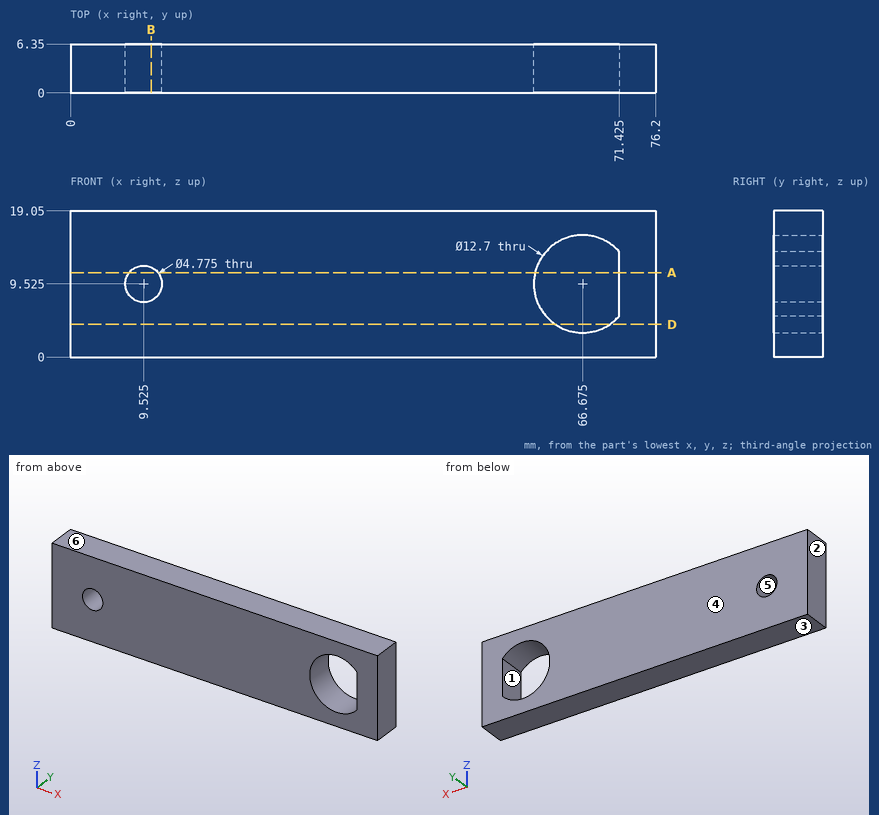
Design review of the part shown in the three views and the two pictorial views. Dimensions are in mm from the part's minimum x, y and z. A direction names the side the tool comes from. Round coordinates to 2 decimals unless told otherwise and drop trailing zeros. Loops run counter-clockwise (first coordinate to the right, second up) from the corner with the lowest first, then second, coordinate; pieces in that order, holes last. Notation, with made-up numbers: (66.25, -8) -> (103.25, -8) arc R23 ccw to (103.25, 11) -> close; hole circle Ø3 at (71.5, 7.25). An arc over 180 degrees is marked (long way). Return JSON: item names as keys, results as strings.
(1) For line 1 (X direction, y = 1.75, z = 9.75) (1 decimal); line 2 (X direction, y = 3.75, z = 7.5) (1 decimal); line 3 (X direction, y = 2.5, z = 5.75) (1 decimal), list the stretches that pass through material, from the lowest coordinate up.
Solved:
{"line 1": "0 to 7.1, 11.9 to 60.3, 71.4 to 76.2", "line 2": "0 to 8.3, 10.8 to 60.7, 71.4 to 76.2", "line 3": "0 to 61.6, 71.4 to 76.2"}
(2) Add section B-B on x = 10.5. Write out the cut boundary in (y, z), plus the area to 3 significant figures.
Solved:
{"outline": "(0, 0) -> (6.35, 0) -> (6.35, 7.35) -> (0, 7.35) -> close; (0, 11.7) -> (6.35, 11.7) -> (6.35, 19.05) -> (0, 19.05) -> close", "area": "93.3 mm2"}
(3) The part is to be moulded in two halves that separate along Z. For the marked faces 3, 4, 5 and 6, say which applies: released by +Z, released by -Z, zero draft, split by the parting line, or undercut.
Solved:
{"face 3": "released by -Z", "face 4": "zero draft", "face 5": "undercut", "face 6": "released by +Z"}
(4) Add section A-A on z = 11. State how many separate pieces and enclosed holes the cut face has, plus the area to 3 significant figures.
Solved:
{"separate pieces": "3", "enclosed holes": "0", "area": "391 mm2"}
(5) For the marked faces 1 and 2, list the 3-axis set-ups (+Z, -Z, +X, -X, +Y, -Y) from which the entire face can be reached by the end or side of a thin tool; tool diameter is ignored.
Solved:
{"face 1": "+Y, -Y", "face 2": "+Z, -Z, -X, +Y, -Y"}
(6) Add section D-D on z = 4.25. Write out the cut boundary in (x, y).
Solved:
{"outline": "(0, 0) -> (63.14, 0) -> (63.14, 6.35) -> (0, 6.35) -> close; (70.21, 0) -> (76.2, 0) -> (76.2, 6.35) -> (70.21, 6.35) -> close"}
(7) For pin 1 (2 mm diameter, centred on y = 1, z = 5, fed in from -X), flat-tipped, find the tip position at first contact; note if it passes through.
Solved:
{"pin 1": "x = 0"}
